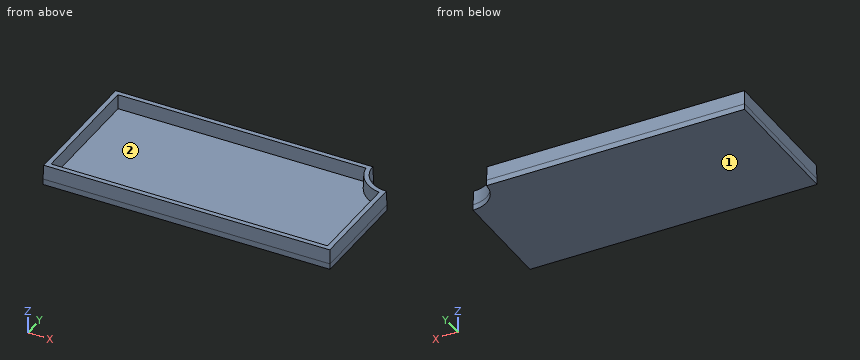
```python
from build123d import *

# Parameters (mm, degrees)
BOSS_EXTRU_1_DEPTH = 2
BOSS_EXTRU_2_DEPTH = 5
BOSS_EXTRU_2_DRAFT = 2


with BuildPart() as part:
    # Esquisse1 → Boss.-Extru.1 (new body)
    with BuildSketch(Plane.XY):
        with BuildLine():
            Line((0, 0), (99.5, 0))
            Line((99.5, 0), (99.5, 37))
            ThreePointArc((99.5, 37), (92.428932188, 39.928932188), (89.5, 47))
            Line((89.5, 47), (0, 47))
            Line((0, 47), (0, 0))
        make_face()
    extrude(amount=BOSS_EXTRU_1_DEPTH)


with BuildPart() as boss_extru_2_tool:
    # Esquisse2 → Boss.-Extru.2 (with draft: the straight prism first)
    with BuildSketch(Plane.XY.offset(2)):
        with BuildLine():
            Line((0, 47), (0, 0))
            Line((0, 0), (99.5, 0))
            Line((99.5, 0), (99.5, 37))
            ThreePointArc((99.5, 37), (92.428932188, 39.928932188), (89.5, 47))
            Line((89.5, 47), (0, 47))
        make_face()
        with BuildLine():
            Line((2, 45), (2, 2))
            Line((2, 2), (97.5, 2))
            Line((97.5, 2), (97.5, 35.167840434))
            ThreePointArc((97.5, 35.167840434), (91.014718626, 38.514718626), (87.667840434, 45))
            Line((87.667840434, 45), (2, 45))
        make_face(mode=Mode.SUBTRACT)
    extrude(amount=BOSS_EXTRU_2_DEPTH)
    # Boss.-Extru.2: the draft: its side faces are tilted about the plane it starts from
    boss_extru_2_sides = [boss_extru_2_tool.faces().sort_by_distance(p)[0] for p in [
        (92.428932188, 39.928932188, 4.5),
        (44.75, 47, 4.5),
        (0, 23.5, 4.5),
        (49.75, 0, 4.5),
        (99.5, 18.5, 4.5),
        (44.833920217, 45, 4.5),
        (91.014718626, 38.514718626, 4.5),
        (97.5, 18.583920217, 4.5),
        (49.75, 2, 4.5),
        (2, 23.5, 4.5),
    ]]
    draft(boss_extru_2_sides, Plane.XY.offset(2), BOSS_EXTRU_2_DRAFT)


with BuildPart() as part_1:
    add(part.part)

    # Boss.-Extru.2: add boss_extru_2_tool
    add(boss_extru_2_tool.part)


solid = part_1.part
```
The listing builds one solid part. Answer for the finished solid, in the listing's coordinates (mm). Face numbers are marked on the shaded views. Give positions to 0.01 mm unless a question says otherwise; leave off trailing zeros. Order: outer loops, then holes, each group sorted by start corner. A loop starts at its lowest first (then second) coordinate and runs counter-clockwise, first axis right, second up.
Item 1: The part is cut by section C-C, the plane z = 5. Give the vertices of the cut face in (x, y).
From the geometry:
outline: (0.1, 0.1) - (99.4, 0.1) - (99.4, 36.9) arc R10.1 cw to (89.4, 46.9) - (0.1, 46.9) - close; hole (1.9, 1.9) - (97.6, 1.9) - (97.6, 35.26) arc R11.9 cw to (87.76, 45.1) - (1.9, 45.1) - close
Item 2: For a pull along Y with two mould halves and no side action, classify the marked faces 1 and 2 as pulls with the +Y half, pulls with the -Y half, needs draft (parallel to the pull), parting line crosses it, or undercut.
From the geometry:
face 1: needs draft
face 2: undercut
Item 3: The part is cut by section B-B, the plane y = 25.5. Give the vertices of the cut face in (x, z), and give its area (3 significant figures).
From the geometry:
outline: (0, 0) - (99.5, 0) - (99.5, 2) - (99.33, 7) - (97.67, 7) - (97.5, 2) - (2, 2) - (1.83, 7) - (0.17, 7) - (0, 2) - close
area: 217 mm2
Item 4: Given pin 1 Ø21.5 at (x, y) = (43, 27) entering from +Z; pin 2 Ø4 at (y, z) = (40, 3.5) entering from -X, each flat-ended and moving along its own axis, determine where each tip first touches the part or whether it passes through.
From the geometry:
pin 1: stops at z = 2
pin 2: stops at x = 0
Item 5: Find the intervals of material crossed by probe 1 along Y at (x, z) = (59.5, 2.5); probe 2 along Y at (x, z) = (50, 6.5); probe 3 along Z at (x, y) = (55.5, 15), in increasing order.
From the geometry:
probe 1: y = 0.02 to 1.98, 45.02 to 46.98
probe 2: y = 0.16 to 1.84, 45.16 to 46.84
probe 3: z = 0 to 2
Item 6: The part is cut by section A-A, the plane x = 23. Give the vertices of the cut face in (y, z).
From the geometry:
outline: (0, 0) - (47, 0) - (47, 2) - (46.83, 7) - (45.17, 7) - (45, 2) - (2, 2) - (1.83, 7) - (0.17, 7) - (0, 2) - close
